Source: CAD feature listing. Evaluate the final solid. Frame: model axes, mm. A direction names the side the tool comes from. Coordinates: 2 decimals unless noted, no trailing zeros. Write each loop counter-clockwise with the first axis right and the second up, starting at its lowest first coordinate (ties: lowest second). Pieces come first, ordered by that corner, then holes. Notation, with made-up numbers: (32, 72.5) -> (76, 72.5) arc R21 ccw to (76, 106.5) -> close; hole circle Ø8 at (77, 27.5). An arc over 180 degrees is marked (long way). One line per item, written item: value. Start each with the question number.
1. First-contact query: P1, Ø12, axis at y = 79.5, z = 220, coming from the +X side. Flat tip, straight axial feed; report the tip coordinate or a pass-through.
2. Line query: line 1 (Z direction, x = 57.5, y = 10); line 2 (X direction, y = 16, z = 251.5); line 3 (Z direction, x = -213, y = 107). Output: solid intervals per line, ascending.
3. Section query D-D, the plane z = 333. Output: boundary loops of the cut face in (x, y), and give its area (3 significant figures).
4. Section query C-C, the plane x = 226.5. Output: boundary loops of the cut face in (y, z), and give its area (3 significant figures).
5. Section query A-A, the plane x = -31. Output: boundary loops of the cut face in (y, z).
6. Section query B-B, the plane z = 15.5. Output: boundary loops of the cut face in (x, y), and give its area (3 significant figures).
7. Access query for faces 3 (the flat face through (-252.941, 59, 372)), 4 (the flat face through (297, 59, 241.922)), 5 (the flat face through (-252.941, 10, 112)). Directions: +Z, -Z, +X, -X, +Y, -Y. A direction counts if a zero-diameter tool reaches every point of the face in a straight line with its end or side. Return the directions, or none.
8. Mould query, pull axis X, two halves, no side actions, for faces 1 (the flat face through (-252.941, 59, -148)), 2 (the flat face through (-263, 59, -138.078)). Classes: released by +X, released by -X, zero draft, split by the parting line, or undercut.
from build123d import *

# Parameters (mm, degrees)
SKETCH_2_W           = 580
SKETCH_2_H           = 540
EXTRUDE_1_DEPTH      = 20
SKETCH_3_W           = 235
SKETCH_3_H           = 200
CUT_EXTRUDE_1_DEPTH  = 21
SKETCH_4_W           = 235
SKETCH_4_H           = 200
CUT_EXTRUDE_2_DEPTH  = 21
SKETCH_5_W           = 235
SKETCH_5_H           = 200
CUT_EXTRUDE_3_DEPTH  = 21
SKETCH_6_W           = 235
SKETCH_6_H           = 200
CUT_EXTRUDE_4_DEPTH  = 21
SKETCH_7_W           = 30
SKETCH_7_H           = 500
CUT_EXTRUDE_5_DEPTH  = 21
SKETCH_8_W           = 235
SKETCH_8_H           = 60
CUT_EXTRUDE_6_DEPTH  = 21
SKETCH_9_W           = 235
SKETCH_9_H           = 60
CUT_EXTRUDE_7_DEPTH  = 21
SKETCH_10_W          = 180
SKETCH_10_H          = 20
EXTRUDE_2_DEPTH      = 100
SKETCH_11_W          = 140
SKETCH_11_H          = 80
CUT_EXTRUDE_8_DEPTH  = 21
SKETCH_12_W          = 20
SKETCH_12_H          = 140
EXTRUDE_3_DEPTH      = 100
SKETCH_13_W          = 120
SKETCH_13_H          = 80
CUT_EXTRUDE_9_DEPTH  = 21
SKETCH_14_W          = 180
SKETCH_14_H          = 20
EXTRUDE_4_DEPTH      = 100
SKETCH_15_W          = 140
SKETCH_15_H          = 80
CUT_EXTRUDE_10_DEPTH = 21
SKETCH_17_W          = 20
SKETCH_17_H          = 160
EXTRUDE_5_DEPTH      = 100
SKETCH_18_W          = 140
SKETCH_18_H          = 80
CUT_EXTRUDE_11_DEPTH = 21
SKETCH_19_W          = 180
SKETCH_19_H          = 20
EXTRUDE_6_DEPTH      = 100
SKETCH_20_W          = 140
SKETCH_20_H          = 80
CUT_EXTRUDE_12_DEPTH = 21
SKETCH_22_W          = 20
SKETCH_22_H          = 140
EXTRUDE_7_DEPTH      = 100
SKETCH_23_W          = 120
SKETCH_23_H          = 80
CUT_EXTRUDE_13_DEPTH = 581
SKETCH_24_W          = 180
SKETCH_24_H          = 20
EXTRUDE_8_DEPTH      = 100
SKETCH_25_W          = 140
SKETCH_25_H          = 80
CUT_EXTRUDE_14_DEPTH = 100
SKETCH_26_W          = 20
SKETCH_26_H          = 140
EXTRUDE_9_DEPTH      = 100
SKETCH_27_W          = 120
SKETCH_27_H          = 80
CUT_EXTRUDE_15_DEPTH = 100


with BuildPart() as part:
    # 草图2 → 凸台-拉伸1 (new body)
    with BuildSketch(Plane(origin=(0, 0, 0), x_dir=(1, 0, 0), z_dir=(0, 1, 0))):
        with Locations((17.058823529, -111.921568627)):
            Rectangle(SKETCH_2_W, SKETCH_2_H)
    extrude(amount=EXTRUDE_1_DEPTH)

    # 草图3 → 切除-拉伸1 (cut, through all)
    with BuildSketch(Plane(origin=(0, 20, 0), x_dir=(1, 0, 0), z_dir=(0, 1, 0))):
        with Locations((-135.441176471, 38.078431373)):
            Rectangle(SKETCH_3_W, SKETCH_3_H)
    extrude(amount=-CUT_EXTRUDE_1_DEPTH, mode=Mode.SUBTRACT)

    # 草图4 → 切除-拉伸2 (cut, through all)
    with BuildSketch(Plane(origin=(0, 20, 0), x_dir=(1, 0, 0), z_dir=(0, 1, 0))):
        with Locations((169.558823529, 38.078431373)):
            Rectangle(SKETCH_4_W, SKETCH_4_H)
    extrude(amount=-CUT_EXTRUDE_2_DEPTH, mode=Mode.SUBTRACT)

    # 草图5 → 切除-拉伸3 (cut, through all)
    with BuildSketch(Plane(origin=(0, 20, 0), x_dir=(1, 0, 0), z_dir=(0, 1, 0))):
        with Locations((-135.441176471, -261.921568627)):
            Rectangle(SKETCH_5_W, SKETCH_5_H)
    extrude(amount=-CUT_EXTRUDE_3_DEPTH, mode=Mode.SUBTRACT)

    # 草图6 → 切除-拉伸4 (cut, through all)
    with BuildSketch(Plane(origin=(0, 20, 0), x_dir=(1, 0, 0), z_dir=(0, 1, 0))):
        with Locations((169.558823529, -261.921568627)):
            Rectangle(SKETCH_6_W, SKETCH_6_H)
    extrude(amount=-CUT_EXTRUDE_4_DEPTH, mode=Mode.SUBTRACT)

    # 草图7 → 切除-拉伸5 (cut, through all)
    with BuildSketch(Plane(origin=(0, 20, 0), x_dir=(1, 0, 0), z_dir=(0, 1, 0))):
        with Locations((17.058823529, -111.921568627)):
            Rectangle(SKETCH_7_W, SKETCH_7_H)
    extrude(amount=-CUT_EXTRUDE_5_DEPTH, mode=Mode.SUBTRACT)

    # 草图8 → 切除-拉伸6 (cut, through all)
    with BuildSketch(Plane(origin=(0, 20, 0), x_dir=(1, 0, 0), z_dir=(0, 1, 0))):
        with Locations((-135.441176471, -111.921568627)):
            Rectangle(SKETCH_8_W, SKETCH_8_H)
    extrude(amount=-CUT_EXTRUDE_6_DEPTH, mode=Mode.SUBTRACT)

    # 草图9 → 切除-拉伸7 (cut, through all)
    with BuildSketch(Plane(origin=(0, 20, 0), x_dir=(1, 0, 0), z_dir=(0, 1, 0))):
        with Locations((169.558823529, -111.921568627)):
            Rectangle(SKETCH_9_W, SKETCH_9_H)
    extrude(amount=-CUT_EXTRUDE_7_DEPTH, mode=Mode.SUBTRACT)

    # 草图10 → 凸台-拉伸2 (add)
    with BuildSketch(Plane(origin=(0, 20, 0), x_dir=(1, 0, 0), z_dir=(0, 1, 0))):
        with Locations((-182.941176471, 148.078431373)):
            Rectangle(SKETCH_10_W, SKETCH_10_H)
    extrude(amount=EXTRUDE_2_DEPTH)

    # 草图11 → 切除-拉伸8 (cut, through all)
    with BuildSketch(Plane.XY.offset(-138.078431373)):
        with Locations((-182.941176471, 60)):
            Rectangle(SKETCH_11_W, SKETCH_11_H)
    extrude(amount=-CUT_EXTRUDE_8_DEPTH, mode=Mode.SUBTRACT)

    # 草图12 → 凸台-拉伸3 (add)
    with BuildSketch(Plane(origin=(0, 20, 0), x_dir=(1, 0, 0), z_dir=(0, 1, 0))):
        with Locations((-262.941176471, 68.078431373)):
            Rectangle(SKETCH_12_W, SKETCH_12_H)
    extrude(amount=EXTRUDE_3_DEPTH)

    # 草图13 → 切除-拉伸9 (cut, through all)
    with BuildSketch(Plane(origin=(-252.941176471, 0, 0), x_dir=(0, 0, -1), z_dir=(1, 0, 0))):
        with Locations((78.078431373, 60)):
            Rectangle(SKETCH_13_W, SKETCH_13_H)
    extrude(amount=-CUT_EXTRUDE_9_DEPTH, mode=Mode.SUBTRACT)

    # 草图14 → 凸台-拉伸4 (add)
    with BuildSketch(Plane(origin=(0, 20, 0), x_dir=(1, 0, 0), z_dir=(0, 1, 0))):
        with Locations((-182.941176471, -371.921568627)):
            Rectangle(SKETCH_14_W, SKETCH_14_H)
    extrude(amount=EXTRUDE_4_DEPTH)

    # 草图15 → 切除-拉伸10 (cut, through all)
    with BuildSketch(Plane(origin=(0, 0, 361.921568627), x_dir=(-1, 0, 0), z_dir=(0, 0, -1))):
        with Locations((182.941176471, 60)):
            Rectangle(SKETCH_15_W, SKETCH_15_H)
    extrude(amount=-CUT_EXTRUDE_10_DEPTH, mode=Mode.SUBTRACT)

    # 草图17 → 凸台-拉伸5 (add)
    with BuildSketch(Plane(origin=(0, 20, 0), x_dir=(1, 0, 0), z_dir=(0, 1, 0))):
        with Locations((-262.941176471, -281.921568627)):
            Rectangle(SKETCH_17_W, SKETCH_17_H)
    extrude(amount=EXTRUDE_5_DEPTH)

    # 草图18 → 切除-拉伸11 (cut, through all)
    with BuildSketch(Plane(origin=(-252.941176471, 0, 0), x_dir=(0, 0, -1), z_dir=(1, 0, 0))):
        with Locations((-291.921568627, 60)):
            Rectangle(SKETCH_18_W, SKETCH_18_H)
    extrude(amount=-CUT_EXTRUDE_11_DEPTH, mode=Mode.SUBTRACT)

    # 草图19 → 凸台-拉伸6 (add)
    with BuildSketch(Plane(origin=(0, 20, 0), x_dir=(1, 0, 0), z_dir=(0, 1, 0))):
        with Locations((217.058823529, 148.078431373)):
            Rectangle(SKETCH_19_W, SKETCH_19_H)
    extrude(amount=EXTRUDE_6_DEPTH)

    # 草图20 → 切除-拉伸12 (cut, through all)
    with BuildSketch(Plane.XY.offset(-138.078431373)):
        with Locations((217.058823529, 60)):
            Rectangle(SKETCH_20_W, SKETCH_20_H)
    extrude(amount=-CUT_EXTRUDE_12_DEPTH, mode=Mode.SUBTRACT)

    # 草图22 → 凸台-拉伸7 (add)
    with BuildSketch(Plane(origin=(0, 20, 0), x_dir=(1, 0, 0), z_dir=(0, 1, 0))):
        with Locations((297.058823529, 68.078431373)):
            Rectangle(SKETCH_22_W, SKETCH_22_H)
    extrude(amount=EXTRUDE_7_DEPTH)

    # 草图23 → 切除-拉伸13 (cut, through all)
    with BuildSketch(Plane(origin=(307.058823529, 0, 0), x_dir=(0, 0, -1), z_dir=(1, 0, 0))):
        with Locations((78.078431373, 60)):
            Rectangle(SKETCH_23_W, SKETCH_23_H)
    extrude(amount=-CUT_EXTRUDE_13_DEPTH, mode=Mode.SUBTRACT)

    # 草图24 → 凸台-拉伸8 (add)
    with BuildSketch(Plane(origin=(0, 20, 0), x_dir=(1, 0, 0), z_dir=(0, 1, 0))):
        with Locations((217.058823529, -371.921568627)):
            Rectangle(SKETCH_24_W, SKETCH_24_H)
    extrude(amount=EXTRUDE_8_DEPTH)

    # 草图25 → 切除-拉伸14 (cut)
    with BuildSketch(Plane(origin=(0, 0, 361.921568627), x_dir=(-1, 0, 0), z_dir=(0, 0, -1))):
        with Locations((-217.058823529, 60)):
            Rectangle(SKETCH_25_W, SKETCH_25_H)
    extrude(amount=-CUT_EXTRUDE_14_DEPTH, mode=Mode.SUBTRACT)

    # 草图26 → 凸台-拉伸9 (add)
    with BuildSketch(Plane(origin=(0, 20, 0), x_dir=(1, 0, 0), z_dir=(0, 1, 0))):
        with Locations((297.058823529, -291.921568627)):
            Rectangle(SKETCH_26_W, SKETCH_26_H)
    extrude(amount=EXTRUDE_9_DEPTH)

    # 草图27 → 切除-拉伸15 (cut)
    with BuildSketch(Plane.ZY.offset(-287.058823529)):
        with Locations((301.921568627, 60)):
            Rectangle(SKETCH_27_W, SKETCH_27_H)
    extrude(amount=-CUT_EXTRUDE_15_DEPTH, mode=Mode.SUBTRACT)


solid = part.part
Computed values:
1. P1: stops at x = 307.06
2. line 1: z = -158.08 to -138.08, 61.92 to 81.92, 141.92 to 161.92, 361.92 to 381.92
2. line 2: x = -272.94 to -252.94, -17.94 to 2.06, 32.06 to 52.06, 287.06 to 307.06
2. line 3: z = -158.08 to -138.08, 361.92 to 381.92
3. outline: (-272.94, 0) -> (-252.94, 0) -> (-252.94, 20) -> (-272.94, 20) -> close; (-272.94, 100) -> (-252.94, 100) -> (-252.94, 120) -> (-272.94, 120) -> close; (-17.94, 0) -> (2.06, 0) -> (2.06, 20) -> (-17.94, 20) -> close; (32.06, 0) -> (52.06, 0) -> (52.06, 20) -> (32.06, 20) -> close; (287.06, 0) -> (307.06, 0) -> (307.06, 20) -> (287.06, 20) -> close; (287.06, 100) -> (307.06, 100) -> (307.06, 120) -> (287.06, 120) -> close
3. area: 2,400 mm²
4. outline: (0, -158.08) -> (20, -158.08) -> (20, -138.08) -> (0, -138.08) -> close; (0, 61.92) -> (20, 61.92) -> (20, 81.92) -> (0, 81.92) -> close; (0, 141.92) -> (20, 141.92) -> (20, 161.92) -> (0, 161.92) -> close; (0, 361.92) -> (20, 361.92) -> (20, 381.92) -> (0, 381.92) -> close; (100, -158.08) -> (120, -158.08) -> (120, -138.08) -> (100, -138.08) -> close; (100, 361.92) -> (120, 361.92) -> (120, 381.92) -> (100, 381.92) -> close
4. area: 2,400 mm²
5. outline: (0, -158.08) -> (20, -158.08) -> (20, -138.08) -> (0, -138.08) -> close; (0, 61.92) -> (20, 61.92) -> (20, 81.92) -> (0, 81.92) -> close; (0, 141.92) -> (20, 141.92) -> (20, 161.92) -> (0, 161.92) -> close; (0, 361.92) -> (20, 361.92) -> (20, 381.92) -> (0, 381.92) -> close
6. outline: (-272.94, 0) -> (-252.94, 0) -> (-252.94, 20) -> (-272.94, 20) -> close; (-17.94, 0) -> (2.06, 0) -> (2.06, 20) -> (-17.94, 20) -> close; (32.06, 0) -> (52.06, 0) -> (52.06, 20) -> (32.06, 20) -> close; (287.06, 0) -> (307.06, 0) -> (307.06, 20) -> (287.06, 20) -> close
6. area: 1,600 mm²
7. face 3: +Z, -Z
7. face 4: +X, -X
7. face 5: +Y, -Y
8. face 1: undercut
8. face 2: zero draft
